Design review of the part shown in the three views and the two pictorial views. Dimensions are in mm from the part's minimum x, y and z. Round coordinates to 2 decimals unless told otherwise and drop trailing zeros. Order: outer loops, then holes, each group sorted by start corner. A loop starts at its lowest first (then second) coordinate and runs counter-clockwise, first axis right, second up. Notation, with made-up numbers: (72.5, -24.75) - (90.5, -24.75) arc R12 cw to (90.5, -3.75) - close; hole circle Ø6 at (-16.75, 15). An arc over 180 degrees is marked (long way). Use CSV: the item, a comma, the result in double quotes.
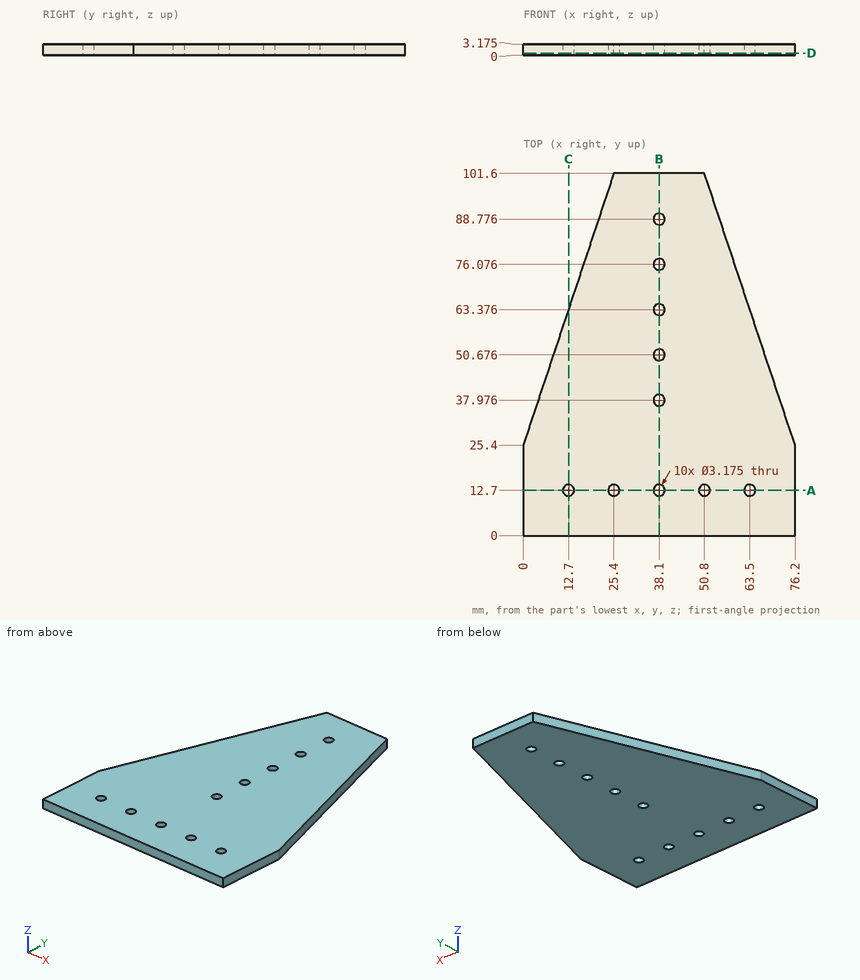
1) We need section A-A (y = 12.7). Give the boundary of the cut face in (x, z) (1 decimal).
Data:
outline,"(0, 0) - (11.1, 0) - (11.1, 3.2) - (0, 3.2) - close; (14.3, 0) - (23.8, 0) - (23.8, 3.2) - (14.3, 3.2) - close; (27, 0) - (36.5, 0) - (36.5, 3.2) - (27, 3.2) - close; (39.7, 0) - (49.2, 0) - (49.2, 3.2) - (39.7, 3.2) - close; (52.4, 0) - (61.9, 0) - (61.9, 3.2) - (52.4, 3.2) - close; (65.1, 0) - (76.2, 0) - (76.2, 3.2) - (65.1, 3.2) - close"
2) We need section C-C (x = 12.7). Give the boundary of the cut face in (y, z) (1 decimal).
Data:
outline,"(0, 0) - (11.1, 0) - (11.1, 3.2) - (0, 3.2) - close; (14.3, 0) - (63.5, 0) - (63.5, 3.2) - (14.3, 3.2) - close"
3) We need section D-D (z = 0.6). Give the number of separate pieces and of enclosed holes in the cut face, then the cut area to 3 significant figures.
Data:
separate pieces,"1"
enclosed holes,"10"
area,"5,730 mm2"
4) We need section B-B (x = 38.1). Give the boundary of the cut face in (y, z) (1 decimal), then the cut area to 3 significant figures.
Data:
outline,"(0, 0) - (11.1, 0) - (11.1, 3.2) - (0, 3.2) - close; (14.3, 0) - (36.4, 0) - (36.4, 3.2) - (14.3, 3.2) - close; (39.6, 0) - (49.1, 0) - (49.1, 3.2) - (39.6, 3.2) - close; (52.3, 0) - (61.8, 0) - (61.8, 3.2) - (52.3, 3.2) - close; (65, 0) - (74.5, 0) - (74.5, 3.2) - (65, 3.2) - close; (77.7, 0) - (87.2, 0) - (87.2, 3.2) - (77.7, 3.2) - close; (90.4, 0) - (101.6, 0) - (101.6, 3.2) - (90.4, 3.2) - close"
area,"262 mm2"
5) To check wall thickness, follow L1, parallel to Y at x = 49.5, z = 1.5; L2, parallel to X at y = 41, z = 0.4; L3, parallel to X at y = 43.5, z = 1.8. State the ranges of each line that lie inside material, in increasing order. Write a range as from..to.
Data:
L1,"y = 0..11.79, 13.61..101.6"
L2,"x = 5.2..71"
L3,"x = 6.03..70.17"
